Here's how the part is built. I have some questions about the finished solid (model axes, mm). Face numbers are marked on the shaded views. Coordinates: 2 decimals unless noted, no trailing zeros.
Item 1: If I drill on line 1 (Z direction, x = 0, y = 12.75); line 2 (X direction, y = 5.5, z = 0); line 3 (X direction, y = 16.25, z = -14), over which ranges is the centre line in solid material (lowest first)?
Item 2: If we section it at A-A (x = 0): Count the separate pieces of the cut face and the enclosed holes in it, then the cut area to 3 significant figures.
Item 3: I'm going to push flat-ended pins straight in: pin 1 Ø8 at (y, z) = (8, -37) entering from +X; pin 2 Ø1 at (x, z) = (-40, 32.5) entering from +Y; pin 3 Ø8 at (y, z) = (3, -24) entering from +X. Where does each tip first touch, or does it pass through?
Item 4: We'd pull the mould along Y, two halves only. Please class the marked faces 1 and 2: +Y half, -Y half, draft (parallel to the pull), parting line (faces both ways), or undercut.
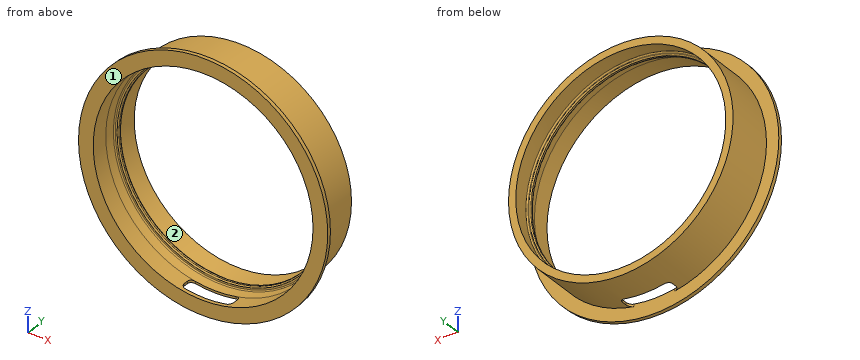
from build123d import *

# Parameters (mm, degrees)
CUT_EXTRUDE1_REACH      = 79.324
CUT_EXTRUDE1_END_RADIUS = 47.3
SKETCH4_W               = 21
SKETCH4_H               = 6
FILLET1_R               = 2
FILLET2_R               = 0.5


with BuildPart() as part:
    # Sketch2 → Revolve1 (revolve)
    with BuildSketch(Plane.XY):
        Polygon((46.3, 0), (46.3, 21.6), (47.3, 21.6), (47.3, 1.6), (52.5, 1.6), (52.5, 0), align=None)
    revolve(axis=Axis((0, -1000, 0), (0, 1, 0)))

    # Cut-Extrude1: up to this cylinder (the profile starts inside it)
    cut_extrude1_end = Plane(origin=(0, 4.6, 0), z_dir=(0, -1, 0)) * Cylinder(CUT_EXTRUDE1_END_RADIUS, 254.248, mode=Mode.PRIVATE)
    # Sketch4 → Cut-Extrude1 (cut, up to the surface)
    with BuildSketch(Plane.XY, mode=Mode.PRIVATE) as cut_extrude1_sk1:
        with Locations((0, 4.6)):
            Rectangle(SKETCH4_W, SKETCH4_H)
    cut_extrude1_tool1 = extrude(cut_extrude1_sk1.sketch, amount=-CUT_EXTRUDE1_REACH, mode=Mode.PRIVATE) & cut_extrude1_end
    add(cut_extrude1_tool1.solids().sort_by_distance((0, 4.6, 0))[0], mode=Mode.SUBTRACT)

    # Fillet1
    fillet1_edges = [part.edges().sort_by_distance(p)[0] for p in [
        (10.5, 1.6, -45.606762076),
        (-10.5, 7.6, -45.606762076),
        (10.5, 7.6, -45.606762076),
        (-10.5, 1.6, -45.606762076),
    ]]
    fillet(fillet1_edges, radius=FILLET1_R)

    # Sketch6 → Revolve2 (revolve)
    with BuildSketch(Plane.XY, mode=Mode.PRIVATE) as revolve2_sk:
        Polygon((-46.3, 7.5), (-44.243032454, 21.6), (-46.3, 21.6), align=None)
        Polygon((-45.431988872, 13.45), (-45.687286263, 11.7), (-44, 11.7), (-44, 13.45), align=None)
    revolve(revolve2_sk.sketch.rotate(Axis((0, -1000, 0), (0, 1, 0)), 180), axis=Axis((0, -1000, 0), (0, 1, 0)))

    # Fillet2
    fillet2_edges = [part.edges().sort_by_distance(p)[0] for p in [
        (-45.687286263, 11.7, 0),
        (-44, 11.7, 0),
        (-44, 13.45, 0),
        (-45.431988872, 13.45, 0),
    ]]
    fillet(fillet2_edges, radius=FILLET2_R)


solid = part.part
Answer list:
1. line 1: z = -47.3 to -44, 44 to 47.3
1. line 2: x = -47.3 to -46.3, 46.3 to 47.3
1. line 3: x = -45.18 to -42.79, 42.79 to 45.18
2. separate pieces: 3
2. enclosed holes: 0
2. area: 88.3 mm2
3. pin 1: stops at x = 33.89
3. pin 2: stops at y = 1.6
3. pin 3: stops at x = 48.44
4. face 1: -Y half
4. face 2: undercut
